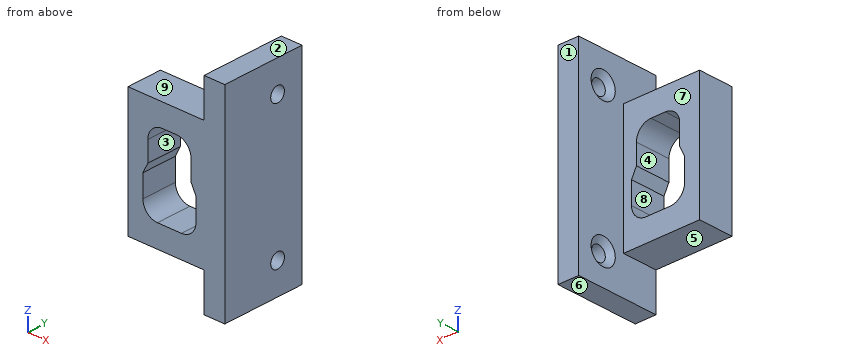
from build123d import *

# Parameters (mm, degrees)
SKETCH1_W                       = 15.24
SKETCH1_H                       = 22.86
BOSS_EXTRUDE2_DEPTH             = 6.4008
CUT_EXTRUDE4_DEPTH              = 1
CUT_EXTRUDE4_DEPTH_BACK         = 7.4008
SKETCH7_W                       = 36.576
SKETCH7_H                       = 15.24
BOSS_EXTRUDE3_DEPTH             = 3.81
F_6_32_TAPPED_HOLE1_D           = 2.7051
F_6_32_TAPPED_HOLE1_CSINK_D     = 4.7752
F_6_32_TAPPED_HOLE1_CSINK_ANGLE = 100


with BuildPart() as part:
    # Sketch1 → Boss-Extrude2 (new body)
    with BuildSketch(Plane(origin=(0, 0, 0), x_dir=(1, 0, 0), z_dir=(0, 1, 0))):
        Rectangle(SKETCH1_W, SKETCH1_H)
        with BuildLine():
            Line((2.208651403, 6.604), (-2.208651403, 6.604))
            ThreePointArc((-2.208651403, 6.604), (-3.555689822, 6.046038418), (-4.113651403, 4.699))
            Line((-4.113651403, 4.699), (-4.113651403, 0.89281026))
            Line((-4.113651403, 0.89281026), (-3.2131, -0.89281026))
            Line((-3.2131, -0.89281026), (-3.2131, -4.699))
            ThreePointArc((-3.2131, -4.699), (-2.655138418, -6.046038418), (-1.3081, -6.604))
            Line((-1.3081, -6.604), (0, -6.604))
            Line((0, -6.604), (1.3081, -6.604))
            ThreePointArc((1.3081, -6.604), (2.655138418, -6.046038418), (3.2131, -4.699))
            Line((3.2131, -4.699), (3.2131, -0.89281026))
            Line((3.2131, -0.89281026), (4.113651403, 0.89281026))
            Line((4.113651403, 0.89281026), (4.113651403, 4.699))
            ThreePointArc((4.113651403, 4.699), (3.555689822, 6.046038418), (2.208651403, 6.604))
        make_face(mode=Mode.SUBTRACT)
    extrude(amount=BOSS_EXTRUDE2_DEPTH)

    # Sketch6 → Cut-Extrude4 (cut, two sides)
    with BuildSketch(Plane(origin=(0, 6.4008, 0), x_dir=(1, 0, 0), z_dir=(0, 1, 0))) as cut_extrude4_sk:
        with BuildLine():
            Line((-3.9751, -1.074087237), (-3.9751, -4.699))
            ThreePointArc((-3.9751, -4.699), (-3.193953785, -6.584853785), (-1.3081, -7.366))
            Line((-1.3081, -7.366), (1.3081, -7.366))
            ThreePointArc((1.3081, -7.366), (3.193953785, -6.584853785), (3.9751, -4.699))
            Line((3.9751, -4.699), (3.9751, -1.074087237))
            Line((3.9751, -1.074087237), (4.875651403, 0.711533282))
            Line((4.875651403, 0.711533282), (4.875651403, 4.699))
            ThreePointArc((4.875651403, 4.699), (4.094505189, 6.584853785), (2.208651403, 7.366))
            Line((2.208651403, 7.366), (-2.208651403, 7.366))
            ThreePointArc((-2.208651403, 7.366), (-4.094505189, 6.584853785), (-4.875651403, 4.699))
            Line((-4.875651403, 4.699), (-4.875651403, 0.711533282))
            Line((-4.875651403, 0.711533282), (-3.9751, -1.074087237))
        make_face()
    extrude(amount=CUT_EXTRUDE4_DEPTH, mode=Mode.SUBTRACT)
    extrude(cut_extrude4_sk.sketch, amount=-CUT_EXTRUDE4_DEPTH_BACK, mode=Mode.SUBTRACT)

    # Sketch7 → Boss-Extrude3 (add)
    with BuildSketch(Plane(origin=(6.35, 0, 0), x_dir=(0, 0, -1), z_dir=(1, 0, 0))):
        with Locations((0, 7.62)):
            Rectangle(SKETCH7_W, SKETCH7_H)
    extrude(amount=BOSS_EXTRUDE3_DEPTH)

    # #6-32 Tapped Hole1 (through all)
    with Locations(Plane.ZY.offset(-6.35)):
        with Locations((12.7, 10.414), (-12.7, 10.414)):
            CounterSinkHole(F_6_32_TAPPED_HOLE1_D / 2, F_6_32_TAPPED_HOLE1_CSINK_D / 2, counter_sink_angle=F_6_32_TAPPED_HOLE1_CSINK_ANGLE)


solid = part.part
Model file for the job. Use its own axes, mm. Face numbers are marked on the shaded views. A direction names the side the tool comes from. Give positions to 0.01 mm unless a question says otherwise; leave off trailing zeros. Order: outer loops, then holes, each group sorted by start corner. A loop starts at its lowest first (then second) coordinate and runs counter-clockwise, first axis right, second up. Notation, with made-up numbers: (79.25, -2) - (124.25, -2) arc R14 cw to (124.25, 25) - close; hole circle Ø7 at (-21, -28). An arc over 180 degrees is marked (long way). Write item = value, one per line. Start each with the question number.
1. Cut at A-A, the plane z = -12.7. List the corners of the cut face in (x, y).
2. Probe line 1 along Z through (x, y) = (0.75, 3); line 2 along Y through (x, z) = (8.3, -12.7); line 3 along Z through (x, y) = (9.25, 9.25). List the from-to ranges inside material, lowest first.
3. Drop flat-ended pins along their axis: P1, Ø5, axis at x = -3, z = -12, coming from the +Y side; P2, Ø3, axis at x = -0.5, y = 3, coming from the -Z side; P3, Ø5, axis at x = -0.5, y = 2, coming from the +Z side. Give the stop position or say it passes through.
4. Cut at D-D, the plane z = -6.5. List the corners of the cut face in (x, y).
5. Cut at C-C, the plane z = 8. List the corners of the cut face in (x, y).
6. Two-plate mould, pull along Z, no slides. Class the marked faces 1, 2, 3 and 4: pulls with the +Z half, pulls with the -Z half, needs draft (parallel to the pull), parting line crosses it, or undercut.
7. Which spindle directions (+Z, -Z, +X, -X, +Y, -Y) get a long thin tool onto all of the face, cutting with end or side? Do the marked faces 5, 6, 7, 8 and 9. Say none if no direction does.
8. Cut at B-B, the plane y = 4.25. List the corners of the cut face in (x, z).
Taken from the geometry:
q1.outline = (6.35, 0) - (10.16, 0) - (10.16, 9.06) - (7.22, 9.06) - (6.35, 8.03) - close; (6.35, 12.8) - (7.22, 11.77) - (10.16, 11.77) - (10.16, 15.24) - (6.35, 15.24) - close
q2.line_1 = -11.43 to -7.37, 7.37 to 11.43
q2.line_2 = 0 to 9.06, 11.77 to 15.24
q2.line_3 = -18.29 to -13.39, -12.01 to 12.01, 13.39 to 18.29
q3.P1 = 6.4
q3.P2 = -11.43
q3.P3 = 11.43
q4.outline = (-7.62, 0) - (-4.18, 0) - (-4.18, 6.4) - (-7.62, 6.4) - close; (4.18, 0) - (10.16, 0) - (10.16, 15.24) - (6.35, 15.24) - (6.35, 6.4) - (4.18, 6.4) - close
q5.outline = (-7.62, 0) - (10.16, 0) - (10.16, 15.24) - (6.35, 15.24) - (6.35, 6.4) - (-7.62, 6.4) - close
q6.face_1 = needs draft
q6.face_2 = pulls with the +Z half
q6.face_3 = undercut
q6.face_4 = undercut
q7.face_5 = -Z, -X, +Y, -Y
q7.face_6 = -Z, +X, -X, +Y, -Y
q7.face_7 = +Z, -Z, -X, +Y
q7.face_8 = +Y, -Y
q7.face_9 = +Z, -X, +Y, -Y
q8.outline = (-7.62, -11.43) - (6.35, -11.43) - (6.35, -18.29) - (10.16, -18.29) - (10.16, 18.29) - (6.35, 18.29) - (6.35, 11.43) - (-7.62, 11.43) - close; hole (-4.88, -4.7) arc R2.67 ccw to (-2.21, -7.37) - (2.21, -7.37) arc R2.67 ccw to (4.88, -4.7) - (4.88, -0.71) - (3.98, 1.07) - (3.98, 4.7) arc R2.67 ccw to (1.31, 7.37) - (-1.31, 7.37) arc R2.67 ccw to (-3.98, 4.7) - (-3.98, 1.07) - (-4.88, -0.71) - close
